CAD build for the part. Positions are in the model's coordinates, mm. A direction names the side the tool comes from. Give positions to 0.01 mm unless a question says otherwise; leave off trailing zeros. Write each loop counter-clockwise with the first axis right and the second up, starting at its lowest first coordinate (ties: lowest second). Pieces come first, ordered by that corner, then holes. Notation, with made-up numbers: (-26.5, 66) - (-20.5, 66) arc R3 cw to (-20.5, 70) - close; hole circle Ø11 at (84, -37.75). An arc over 180 degrees is marked (long way). Answer as a JSON object with one key per item and string values.
from build123d import *

# Parameters (mm, degrees)
F0_W      = 101.6
F0_H      = 101.599996
F1_DEPTH  = 76.2
F2_W      = 88.9
F2_H      = 88.9
F3_DEPTH  = 69.85
F4_W      = 76.2
F4_H      = 57.15
F5_DEPTH  = 12.7
F6_W      = 76.2
F6_H      = 50.8
F7_DEPTH  = 1.27
F8_W      = 76.2
F8_H      = 50.8
F9_DEPTH  = 1.27
F10_W     = 76.2
F10_H     = 50.8
F11_DEPTH = 1.27
F12_W     = 101.6
F12_H     = 177.8
F13_DEPTH = 6.35


with BuildPart() as f1:
    # F0 (on Top) → F1 (new body)
    with BuildSketch(Plane.XY):
        with Locations((4.893579, -0.244679)):
            Rectangle(F0_W, F0_H)
    extrude(amount=F1_DEPTH)

    # F2 (on face) → F3 (cut)
    with BuildSketch(Plane.XY.offset(76.2)):
        with Locations((4.812017, -0.163119)):
            Rectangle(F2_W, F2_H)
    extrude(amount=-F3_DEPTH, mode=Mode.SUBTRACT)

    # F4 (on face) → F5 (cut)
    with BuildSketch(Plane.XZ.offset(51.044677)):
        with Locations((5.06835, 34.925)):
            Rectangle(F4_W, F4_H)
    extrude(amount=-F5_DEPTH, mode=Mode.SUBTRACT)

    # F6 (on face) → F7 (cut)
    with BuildSketch(Plane(origin=(-45.906421, 0, 0), x_dir=(0, -1, 0), z_dir=(-1, 0, 0))):
        with Locations((0.071097, 38.046492)):
            Rectangle(F6_W, F6_H)
    extrude(amount=-F7_DEPTH, mode=Mode.SUBTRACT)

    # F8 (on face) → F9 (cut)
    with BuildSketch(Plane(origin=(0, 50.555319, 0), x_dir=(-1, 0, 0), z_dir=(0, 1, 0))):
        with Locations((-5.701129, 38.046894)):
            Rectangle(F8_W, F8_H)
    extrude(amount=-F9_DEPTH, mode=Mode.SUBTRACT)

    # F10 (on face) → F11 (cut)
    with BuildSketch(Plane.YZ.offset(55.693579)):
        with Locations((-0.148215, 37.570929)):
            Rectangle(F10_W, F10_H)
    extrude(amount=-F11_DEPTH, mode=Mode.SUBTRACT)

    # F12 (on Top) → F13 (join)
    with BuildSketch(Plane.XY):
        with Locations((4.99807, -38.540878)):
            Rectangle(F12_W, F12_H)
    extrude(amount=-F13_DEPTH)


solid = f1.part
(1) Saw through at A-A, the plane x = -18. Give the cut face in (y, z).
Answer key:
{"outline": "(-127.44, -6.35) - (50.36, -6.35) - (50.36, 0) - (50.56, 0) - (50.56, 12.65) - (49.29, 12.65) - (49.29, 63.45) - (50.56, 63.45) - (50.56, 76.2) - (44.29, 76.2) - (44.29, 6.35) - (-51.04, 6.35) - (-51.04, 0) - (-127.44, 0) - close; (-51.04, 63.5) - (-44.61, 63.5) - (-44.61, 76.2) - (-51.04, 76.2) - close"}
(2) Probe L1, parallel to X at y = -50, z = 31; L2, parallel to X at y = 40, z = 29.5; L3, parallel to Y at x = 38, z = 43. List the from-to ranges inside material, lowest first. Write a range as [from, to].
Answer key:
{"L1": "x = [-45.91, -33.03], [43.17, 55.69]", "L2": "x = [-45.91, -39.64], [49.26, 55.69]", "L3": "y = [44.29, 49.29]"}
(3) Saw through at C-C, the plane z = 48. Give the cut face in (x, y).
Answer key:
{"outline": "(-45.91, -51.04) - (-33.03, -51.04) - (-33.03, -44.61) - (-39.64, -44.61) - (-39.64, 44.29) - (49.26, 44.29) - (49.26, -44.61) - (43.17, -44.61) - (43.17, -51.04) - (55.69, -51.04) - (55.69, -38.25) - (54.42, -38.25) - (54.42, 37.95) - (55.69, 37.95) - (55.69, 50.56) - (43.8, 50.56) - (43.8, 49.29) - (-32.4, 49.29) - (-32.4, 50.56) - (-45.91, 50.56) - (-45.91, 38.03) - (-44.64, 38.03) - (-44.64, -38.17) - (-45.91, -38.17) - close"}
(4) Pull direction X, two halves, no side cores. Call faces 6 (the face through (55.694, -1, 12)), 7 (the face through (49.262, -1, 42)), 8 (the face through (-44.636, 0, 38)): pulls with the +X half, pulls with the -X half, needs draft (parallel to the pull), parting line crosses it, or undercut.
Answer key:
{"face 6": "pulls with the +X half", "face 7": "undercut", "face 8": "pulls with the -X half"}
(5) Saw through at D-D, the plane z = 71. Give the cut face in (x, y), and give its area (3 significant figures).
Answer key:
{"outline": "(-45.91, -51.04) - (55.69, -51.04) - (55.69, 50.56) - (-45.91, 50.56) - close; hole (-39.64, -44.61) - (49.26, -44.61) - (49.26, 44.29) - (-39.64, 44.29) - close", "area": "2,420 mm²"}
(6) Flat gauge pins, fed straight in: P1, Ø10, axis at x = 14.5, z = 52.5, coming from the -Y side; P2, Ø10, axis at x = 39.5, y = -15, coming from the +Z side; P3, Ø6, axis at y = -26.5, z = 53.5, coming from the -X side; P4, Ø10, axis at x = 15.5, z = 14, coming from the +Y side. Where does each tip first touch, or does it go through?
Answer key:
{"P1": "stops at y = 44.29", "P2": "stops at z = 6.35", "P3": "stops at x = -44.64", "P4": "stops at y = 50.56"}
(7) Saw through at B-B, the plane y = -40.5. Give the cut face in (x, z).
Answer key:
{"outline": "(-45.91, 0) - (-45.8, 0) - (-45.8, -6.35) - (55.8, -6.35) - (55.8, 0) - (55.69, 0) - (55.69, 76.2) - (49.26, 76.2) - (49.26, 6.35) - (-39.64, 6.35) - (-39.64, 76.2) - (-45.91, 76.2) - close"}
(8) 3-axis set-ups, long thin cutter, end or side, ignore diameter. For faces 1 (the face through (4, 50.359, -3)), 2 (the face through (43.168, -48, 35)), 3 (the face through (6, 49.285, 38)), 4 (the face through (54.424, -1, 38)), 5 (the face through (4, -127.441, -3)): which of +Z, -Z, +X, -X, +Y, -Y reach the whole face in a straight line?
Answer key:
{"face 1": "-Z, +X, -X, +Y", "face 2": "-Y", "face 3": "+Y", "face 4": "+X", "face 5": "+Z, -Z, +X, -X, -Y"}
